Solid Edge part; units mm, degrees
sketch "Sketch1" plane through (0, 0, 0) normal (0, 0, 1) x (1, 0, 0)
  line L0 (0, 0) -> (228.6, 0)
  line L1 (228.6, 0) -> (228.6, 457.2)
  line L2 (228.6, 457.2) -> (0, 457.2)
  line L3 (0, 457.2) -> (0, 0)
  dimension "D1" = 228.6
extrude "Protrusion1" add sketch "Sketch1" along normal blind 4.4958
hole "Hole_1" at (69.85, 66.675, 4.4958) direction (0, 0, -1) diameter 7.9375 end up to next
hole "Hole1" at (158.75, 66.675, 4.4958) direction (0, 0, -1) diameter 7.9375 end up to next
hole "Hole2" at (158.75, 390.525, 4.4958) direction (0, 0, -1) diameter 7.9375 end up to next
hole "Hole3" at (69.85, 390.525, 4.4958) direction (0, 0, -1) diameter 7.9375 end up to next
fillet "Round_1" radius 25.4 2 edges at (228.6, 457.2, 2.2479) (0, 457.2, 2.2479)
sketch "Sketch2" plane through (114.3, 228.6, 0) normal (0, 0, -1) x (0, -1, 0)
  line L0 (-106.0958, 109.8042) -> (-106.0958, 114.3)
  line L1 (-106.0958, 114.3) -> (-42.5958, 114.3)
  line L2 (-42.5958, 109.8042) -> (-42.5958, 114.3)
  line L3 (-106.0958, 109.8042) -> (-42.5958, 109.8042)
  line L4 (147.9042, 114.3) -> (198.7042, 114.3)
  line L5 (198.7042, 109.8042) -> (198.7042, 114.3)
  line L6 (147.9042, 109.8042) -> (198.7042, 109.8042)
  line L7 (147.9042, 109.8042) -> (147.9042, 114.3)
  line L8 (-4.4958, 109.8042) -> (-4.4958, 114.3)
  line L9 (-4.4958, 114.3) -> (33.6042, 114.3)
  line L10 (33.6042, 109.8042) -> (33.6042, 114.3)
  line L11 (-4.4958, 109.8042) -> (33.6042, 109.8042)
  line L12 (71.7042, 109.8042) -> (71.7042, 114.3)
  line L13 (71.7042, 114.3) -> (109.8042, 114.3)
  line L14 (109.8042, 109.8042) -> (109.8042, 114.3)
  line L15 (71.7042, 109.8042) -> (109.8042, 109.8042)
extrude "Cutout1" cut sketch "Sketch2" against normal through all
mirror "Mirror1" about plane through (114.3, 0, 0) normal (-1, 0, 0) of "Cutout1"
sketch "Sketch3" plane through (114.3, 228.6, 0) normal (0, 0, -1) x (-1, 0, 0)
  line L0 (25.4, -224.1042) -> (-25.4, -224.1042)
  line L1 (-25.4, -224.1042) -> (-25.4, -228.6)
  line L2 (25.4, -228.6) -> (-25.4, -228.6)
  line L3 (25.4, -224.1042) -> (25.4, -228.6)
  line L4 (-76.2, -224.1042) -> (-76.2, -228.6)
  line L5 (-76.2, -228.6) -> (-114.3, -228.6)
  line L6 (-114.3, -224.1042) -> (-114.3, -228.6)
  line L7 (-76.2, -224.1042) -> (-114.3, -224.1042)
  line L8 (76.2, -224.1042) -> (76.2, -228.6)
  line L9 (114.3, -228.6) -> (76.2, -228.6)
  line L10 (114.3, -224.1042) -> (114.3, -228.6)
  line L11 (76.2, -224.1042) -> (114.3, -224.1042)
extrude "Cutout3" cut sketch "Sketch3" against normal through all
properties material "Acrylic, high impact grade"
Build history of the part. All positions in model axes, mm. Give positions to 0.01 mm unless a question says otherwise; leave off trailing zeros. Loops run counter-clockwise (first coordinate to the right, second up) from the corner with the lowest first, then second, coordinate; pieces in that order, holes last.
1) Two-plate mould, pull along Y, no slides. Class faces 1 (the face through (221.36, 449.56, 2.28)), 2 (the face through (113, 232, 4.496)), 3 (the face through (68.33, 386.86, 2.28)), 4 (the face through (159.94, 62.89, 2.28)): released by +Y, released by -Y, zero draft, split by the parting line, or undercut.
Values follow:
face 1: released by +Y
face 2: zero draft
face 3: undercut
face 4: undercut
2) Drop flat-ended pins along their axis: P1, Ø2, axis at x = 2.5, z = 2, coming from the -Y side; P2, Ø2, axis at y = 211, z = 2.5, coming from the +X side; P3, Ø2, axis at x = 227, z = 3, coming from the +Y side. Give the stop position or say it passes through.
Values follow:
P1: stops at y = 4.5
P2: stops at x = 224.1
P3: stops at y = 442.99
3) Band-saw the part on A-A on z = 1.3. State how many separate pieces and enclosed holes the cut face has, then the cut area to 3 significant figures.
Values follow:
separate pieces: 1
enclosed holes: 4
area: 102,000 mm2
4) Band-saw the part on B-B on x = 214. List the corners of the cut face in (y, z).
Values follow:
outline: (4.5, 0) - (454.79, 0) - (454.79, 4.5) - (4.5, 4.5) - close
5) Probe line 1 along Y through (x, z) = (69.5, 1); line 2 along Y through (x, z) = (162, 4.15); line 3 along X through (y, z) = (38, 2.8). List the from-to ranges inside material, lowest first.
Values follow:
line 1: y = 0 to 62.72, 70.63 to 386.57, 394.48 to 457.2
line 2: y = 0 to 64.4, 68.95 to 388.25, 392.8 to 457.2
line 3: x = 4.5 to 224.1
